```python
from build123d import *

# Parameters (mm, degrees)
SKETCH1_R           = 1.5
SKETCH1_W           = 3
SKETCH1_H           = 4
BOSS_EXTRUDE2_DEPTH = 3
FILLET1_R           = 8.464107
SKETCH2_R           = 1
CUT_EXTRUDE1_DEPTH  = 3


with BuildPart() as part:
    # Sketch1 → Boss-Extrude2 (new body)
    with BuildSketch(Plane(origin=(0, 0, 0), x_dir=(1, 0, 0), z_dir=(0, 1, 0))):
        with BuildLine():
            Line((-7.5, -42), (-12.409150917, -1.504318289))
            ThreePointArc((-12.409150917, -1.504318289), (0, 12.5), (12.409150917, -1.504318289))
            Line((12.409150917, -1.504318289), (7.5, -42))
            Line((7.5, -42), (-7.5, -42))
        make_face()
        with Locations(Location((0, 0, 0), (0, 0, 270))):
            Circle(SKETCH1_R, mode=Mode.SUBTRACT)
        with Locations((2.75, -18.9)):
            Rectangle(SKETCH1_W, SKETCH1_H, mode=Mode.SUBTRACT)
        with Locations((-2.75, -18.9)):
            Rectangle(SKETCH1_W, SKETCH1_H, mode=Mode.SUBTRACT)
        with Locations((2.75, -35.1)):
            Rectangle(SKETCH1_W, SKETCH1_H, mode=Mode.SUBTRACT)
        with Locations((-2.75, -35.1)):
            Rectangle(SKETCH1_W, SKETCH1_H, mode=Mode.SUBTRACT)
    extrude(amount=BOSS_EXTRUDE2_DEPTH)

    # Fillet1
    fillet1_edges = [part.edges().sort_by_distance(p)[0] for p in [
        (7.5, 1.5, 42),
        (-7.5, 1.5, 42),
    ]]
    fillet(fillet1_edges, radius=FILLET1_R)

    # Sketch2 → Cut-Extrude1 (cut)
    with BuildSketch(Plane(origin=(0, 3, 0), x_dir=(1, 0, 0), z_dir=(0, 1, 0))):
        with Locations(Location((0, 7, 0), (0, 0, 270))):
            Circle(SKETCH2_R)
        with Locations(Location((4.949747468, 4.949747468, 0), (0, 0, 270))):
            Circle(SKETCH2_R)
        with Locations(Location((7, 0, 0), (0, 0, 270))):
            Circle(SKETCH2_R)
        with Locations(Location((4.949747468, -4.949747468, 0), (0, 0, 270))):
            Circle(SKETCH2_R)
        with Locations(Location((0, -7, 0), (0, 0, 270))):
            Circle(SKETCH2_R)
        with Locations(Location((-4.949747468, -4.949747468, 0), (0, 0, 270))):
            Circle(SKETCH2_R)
        with Locations(Location((-7, 0, 0), (0, 0, 270))):
            Circle(SKETCH2_R)
        with Locations(Location((-4.949747468, 4.949747468, 0), (0, 0, 270))):
            Circle(SKETCH2_R)
    extrude(amount=-CUT_EXTRUDE1_DEPTH, mode=Mode.SUBTRACT)


solid = part.part
```
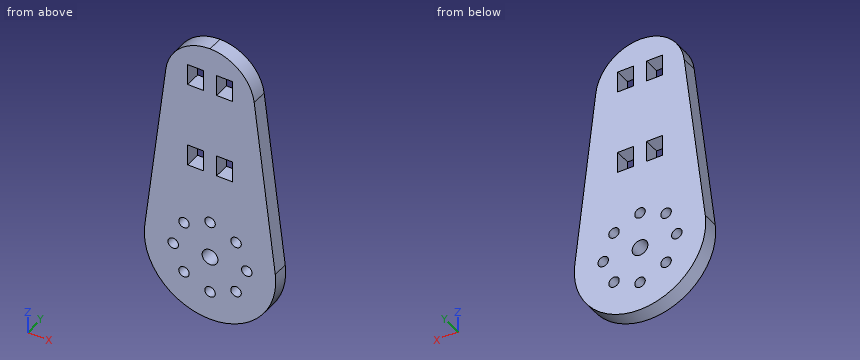
Can you work these out from the model? Positions are in its coordinate system, mm. Coordinates: 2 decimals unless noted, no trailing zeros. Write each loop counter-clockwise with the first axis right and the second up, starting at its lowest first coordinate (ties: lowest second). Pieces come first, ordered by that corner, then holes. Notation, with made-up numbers: (58, 27.5) - (109, 27.5) arc R14 cw to (109, 47.5) - close; hole circle Ø10 at (-6, 47). An arc over 180 degrees is marked (long way). Return JSON: item names as keys, results as strings.
Q1. If we section it at B-B (x = -0.5): Please give me the cut outline in (y, z), then the cut area to 3 significant figures.
Computed values:
{"outline": "(0, -12.49) - (3, -12.49) - (3, -7.87) - (0, -7.87) - close; (0, -6.13) - (3, -6.13) - (3, -1.41) - (0, -1.41) - close; (0, 1.41) - (3, 1.41) - (3, 6.13) - (0, 6.13) - close; (0, 7.87) - (3, 7.87) - (3, 41.99) - (0, 41.99) - close", "area": "145 mm2"}
Q2. Please list where these lines run through material, in increasing order: L1, parallel to X at y = 2.15, z = 0; L2, parallel to Z at x = -2.5, y = 0.8; L3, parallel to Z at x = 3.25, y = 1.95. Write a range as from..to.
Computed values:
{"L1": "x = -12.5..-8, -6..-1.5, 1.5..6, 8..12.5", "L2": "z = -12.25..16.9, 20.9..33.1, 37.1..41.62", "L3": "z = -12.07..16.9, 20.9..33.1, 37.1..41.35"}
Q3. I'm going to push flat-ended pins straight in: pin 1 Ø1.5 at (y, z) = (2, 18.5) entering from +X; pin 2 Ø1.5 at (x, y) = (2.5, 2) entering from -Z; pin 3 Ø1.5 at (x, y) = (-3, 2) entering from -Z. Where does each tip first touch, or does it pass through?
Computed values:
{"pin 1": "stops at x = 10.44", "pin 2": "stops at z = -12.38", "pin 3": "stops at z = -12.3"}
Q4. If we section it at C-C (z = 20): Please give me the cut outline in (x, y).
Computed values:
{"outline": "(-10.17, 0) - (-4.25, 0) - (-4.25, 3) - (-10.17, 3) - close; (-1.25, 0) - (1.25, 0) - (1.25, 3) - (-1.25, 3) - close; (4.25, 0) - (10.17, 0) - (10.17, 3) - (4.25, 3) - close"}
Q5. If we section it at A-A (z = 0): Please give me the cut outline in (x, y), then the cut area to 3 significant figures.
Computed values:
{"outline": "(-12.5, 0) - (-8, 0) - (-8, 3) - (-12.5, 3) - close; (-6, 0) - (-1.5, 0) - (-1.5, 3) - (-6, 3) - close; (1.5, 0) - (6, 0) - (6, 3) - (1.5, 3) - close; (8, 0) - (12.5, 0) - (12.5, 3) - (8, 3) - close", "area": "54.0 mm2"}
Q6. If we section it at D-D (z = 7): Please give me the cut outline in (x, y).
Computed values:
{"outline": "(-11.74, 0) - (-1, 0) - (-1, 3) - (-11.74, 3) - close; (1, 0) - (11.74, 0) - (11.74, 3) - (1, 3) - close"}
